Geometry: final body of the model. Coordinates: model frame, mm. A direction names the side the tool comes from. Coordinates: 2 decimals unless noted, no trailing zeros. Loops run counter-clockwise (first coordinate to the right, second up) from the corner with the lowest first, then second, coordinate; pieces in that order, holes last. Notation, with made-up numbers: (77, -35.75) - (98, -35.75) arc R11 ccw to (98, -24.75) - close; hole circle Ø7 at (35.25, -33). An arc over 180 degrees is marked (long way). Put each result on its own line as item: value. Start each with the question number.
1) Material intervals for line 1 along Y through (x, z) = (5, 1.5); line 2 along X through (y, z) = (29, 109), sorted ascending. Write a range as from..to.
2) Section A-A on z = 68.5. Output: boundary loops of the cut face in (x, y), and give its area (3 significant figures).
3) Contact query for flat-ended pins moving along their axis: pin 1 Ø7 at (x, y) = (5, 5) entering from -Z; pin 2 Ø6 at (x, z) = (40.5, -2) entering from -Y; pin 3 Ø1.5 at (y, z) = (9.5, -3.5) entering from -X; pin 4 Ø6 at (x, y) = (49.5, 38) entering from -Z. Output: stop coordinate, or through.
4) Reachability of faces 5 (the flat face through (24.8, 24.8, -3)), 6 (the cylindrical face through (9.725, 52.111, 65.559)), 7 (the flat face through (52.7, 7.3, 7)) from +Z, -Z, +X, -X, +Y, -Y: full face, straight path, thin tool, end or side. Return the list, or none.
5) Draft query along X for faces 1 (the cylindrical face through (57.182, 53.327, 3.451)), 2 (the cylindrical face through (59.1, 0.86, 3.55)), 3 (the cylindrical face through (35.42, 5.594, -1.479)), 4 (the flat face through (30, 30, -30)). Return one class per face: +X half, -X half, draft (parallel to the pull), parting line (faces both ways), or undercut.
```python
from build123d import *

# Parameters (mm, degrees)
SKETCH_1_W               = 60.00000000000001
SKETCH_1_H               = 60.00000000000001
EXTRUDE_1_DEPTH          = 124.5
SKETCH_2_R               = 25
EXTRUDE_2_DEPTH          = 3
SKETCH_3_R               = 6.999999999999999
EXTRUDE_3_DEPTH          = 27
FILLET_1_R               = 3
CUT_EXTRUDE_1_DEPTH      = 117.5
PATTERN_CIRCULAR_1_COUNT = 4
CHAMFER_1_SIZE           = 2
SKETCH_5_R               = 2.75
SKETCH_5_R_2             = 2.7500000000000018
SKETCH_5_R_3             = 2.7500000000000004
SKETCH_5_R_4             = 2.750000000000002
CUT_EXTRUDE_2_DEPTH      = 151.66602138504885


with BuildPart() as part:
    # 草圖1 → 伸長1 (new body)
    with BuildSketch(Plane.XY):
        with Locations((30.000000000000004, 30.000000000000004)):
            Rectangle(SKETCH_1_W, SKETCH_1_H)
    extrude(amount=EXTRUDE_1_DEPTH)

    # 草圖2 → 伸長2 (add)
    with BuildSketch(Plane(origin=(0, 0, 0), x_dir=(-1, 0, 0), z_dir=(0, 0, -1))):
        with Locations((-30.000000000000007, 30)):
            Circle(SKETCH_2_R)
    extrude(amount=EXTRUDE_2_DEPTH)

    # 草圖3 → 伸長3 (add)
    with BuildSketch(Plane(origin=(0, 0, -3), x_dir=(-1, 0, 0), z_dir=(0, 0, -1))):
        with Locations((-30.000000000000007, 30)):
            Circle(SKETCH_3_R)
    extrude(amount=EXTRUDE_3_DEPTH)

    # 圓角1
    fillet_1_edges = [part.edges().sort_by_distance(p)[0] for p in [
        (0, 60, 62.25),
        (60, 60, 62.25),
        (60, 0, 62.25),
        (0, 0, 62.25),
    ]]
    fillet(fillet_1_edges, radius=FILLET_1_R)

    # 草圖4 → 除料-伸長1 (cut)
    with BuildSketch(Plane.XY.offset(124.5)):
        with BuildLine():
            Line((60, 3), (60, 30.000000000000007))
            ThreePointArc((60, 30.000000000000007), (51.213203435596434, 8.786796564403577), (30, 0))
            Line((30, 0), (56.99999999999999, 0))
            ThreePointArc((56.99999999999999, 0), (59.12132034355964, 0.8786796564403576), (60, 3))
        make_face()
    cut_extrude_1 = extrude(amount=-CUT_EXTRUDE_1_DEPTH, mode=Mode.SUBTRACT)

    # 環狀複製排列1: 除料-伸長1 ×4 about axis
    pattern_circular_1_axis = Axis((30, 30, 0), (0, 0, 1))
    for i in range(1, PATTERN_CIRCULAR_1_COUNT):
        add(cut_extrude_1.rotate(pattern_circular_1_axis, i * 360 / PATTERN_CIRCULAR_1_COUNT), mode=Mode.SUBTRACT)

    # 導角1
    chamfer_1_edges = [part.edges().sort_by_distance(p)[0] for p in [
        (29.999999999999982, 59.99999999999999, 124.5),
    ]]
    chamfer(chamfer_1_edges, length=CHAMFER_1_SIZE)

    # 草圖5 → 除料-伸長2 (cut, through all)
    with BuildSketch(Plane(origin=(0, 0, 0), x_dir=(-1, 0, 0), z_dir=(0, 0, -1))):
        with Locations((-4.999999999999972, 4.999999999999999)):
            Circle(SKETCH_5_R)
        with Locations((-54.99999999999997, 4.999999999999987)):
            Circle(SKETCH_5_R_2)
        with Locations((-4.99999999999997, 54.99999999999999)):
            Circle(SKETCH_5_R_3)
        with Locations((-55, 54.99999999999998)):
            Circle(SKETCH_5_R_4)
    extrude(amount=-CUT_EXTRUDE_2_DEPTH, mode=Mode.SUBTRACT)


solid = part.part
```
Answer block:
1. line 1: y = 0..2.25, 7.75..52.25, 57.75..60
1. line 2: x = 0.02..59.98
2. outline: circle Ø60 at (30, 30)
2. area: 2,830 mm²
3. pin 1: stops at z = 0
3. pin 2: stops at y = 0
3. pin 3: stops at x = 14.92
3. pin 4: stops at z = -3
4. face 5: -Z
4. face 6: +Z
4. face 7: +Z, +X, -Y
5. face 1: undercut
5. face 2: +X half
5. face 3: parting line
5. face 4: draft
